Check sheet for the modelled part. Datum: model origin and axes. Units: mm. Face numbers are marked on the shaded views. A direction names the side the tool comes from. Round coordinates to 2 decimals unless told otherwise and drop trailing zeros. Loops run counter-clockwise (first coordinate to the right, second up) from the corner with the lowest first, then second, coordinate; pieces in that order, holes last. Notation, with made-up numbers: (-27, 22.25) - (-3, 22.25) arc R33 ccw to (-3, 56.25) - close; hole circle Ø4 at (2, 28). An arc over 180 degrees is marked (long way). Put each result on its own line as item: value.
```python
from build123d import *

# Parameters (mm, degrees)
SKETCH1_W           = 25
SKETCH1_H           = 16
BOSS_EXTRUDE1_DEPTH = 1
SKETCH2_W           = 20.55
SKETCH2_H           = 11.8
BOSS_EXTRUDE2_DEPTH = 2
FILLET1_R           = 2.5
FILLET2_R           = 0.5


with BuildPart() as part:
    # Sketch1 → Boss-Extrude1 (new body)
    with BuildSketch(Plane.XY):
        Rectangle(SKETCH1_W, SKETCH1_H)
    extrude(amount=-BOSS_EXTRUDE1_DEPTH)

    # Sketch2 → Boss-Extrude2 (add)
    with BuildSketch(Plane.XY):
        Rectangle(SKETCH2_W, SKETCH2_H)
    extrude(amount=BOSS_EXTRUDE2_DEPTH)

    # Fillet1
    fillet1_edges = [part.edges().sort_by_distance(p)[0] for p in [
        (10.275, -5.9, 1),
        (10.275, 5.9, 1),
        (-10.275, 5.9, 1),
        (-10.275, -5.9, 1),
        (12.5, -8, -0.5),
        (-12.5, -8, -0.5),
        (-12.5, 8, -0.5),
        (12.5, 8, -0.5),
    ]]
    fillet(fillet1_edges, radius=FILLET1_R)

    # Fillet2
    fillet2_edges = [part.edges().sort_by_distance(p)[0] for p in [
        (0, 5.9, 2),
        (10.275, 0, 2),
        (-10.275, 0, 2),
        (0, -5.9, 2),
        (9.542766953, -5.167766953, 2),
        (-9.542766953, -5.167766953, 2),
        (-9.542766953, 5.167766953, 2),
        (9.542766953, 5.167766953, 2),
    ]]
    fillet(fillet2_edges, radius=FILLET2_R)


solid = part.part
```
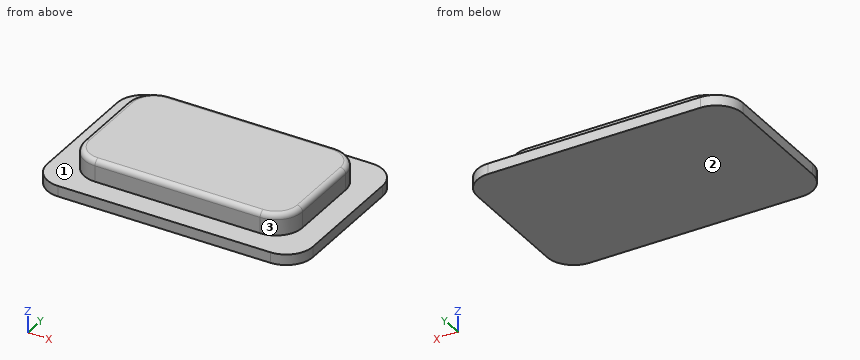
Item 1: Section check C-C on x = -3.25. Enter the section's corners in (y, z).
Filled sheet:
outline: (-8, -1) - (8, -1) - (8, 0) - (5.9, 0) - (5.9, 1.5) arc R0.5 ccw to (5.4, 2) - (-5.4, 2) arc R0.5 ccw to (-5.9, 1.5) - (-5.9, 0) - (-8, 0) - close
Item 2: Thickness scan on line 1 (Z direction, x = 11.25, y = 5.25); line 2 (X direction, y = 1.5, z = 0.3) (3 decimals); line 3 (Y direction, x = 0.75, z = 0.25). Record the ranges inside material, lowest first. Write a range as from..to.
Filled sheet:
line 1: -1..0
line 2: -10.275..10.275
line 3: -5.9..5.9
Item 3: Section check B-B on y = 0. Enter the section's corners in (x, z) (3 decimals), then the cut area to 3 significant figures.
Filled sheet:
outline: (-12.5, -1) - (12.5, -1) - (12.5, 0) - (10.275, 0) - (10.275, 1.5) arc R0.5 ccw to (9.775, 2) - (-9.775, 2) arc R0.5 ccw to (-10.275, 1.5) - (-10.275, 0) - (-12.5, 0) - close
area: 66.0 mm²
Item 4: Section check A-A on z = 0.4. Enter the section's corners in (x, y) (3 decimals).
Filled sheet:
outline: (-10.275, -3.4) arc R2.5 ccw to (-7.775, -5.9) - (7.775, -5.9) arc R2.5 ccw to (10.275, -3.4) - (10.275, 3.4) arc R2.5 ccw to (7.775, 5.9) - (-7.775, 5.9) arc R2.5 ccw to (-10.275, 3.4) - close
Item 5: Tool access check on the marked faces 1, 2 and 3. Record the directions out of +Z, -Z, +X, -X, +Y, -Y that give a thin tool (end or side, any length) a straight path to the whole face; none if there is none.
Filled sheet:
face 1: +Z
face 2: -Z, +X, -X, +Y, -Y
face 3: +Z, +X, -Y
Item 6: Go/stop test with flat-tipped pins: pin 1 (0.8 mm diameter, centred on y = -0.5, z = 1, fed in from -X) (3 decimals); pin 2 (0.8 mm diameter, centred on x = 1.5, z = 1, fed in from -Y); pin 3 (1.2 mm diameter, centred on x = 0, z = 1, fed in from +Y). Record where each tip stops, or that it passes through.
Filled sheet:
pin 1: x = -10.275
pin 2: y = -5.9
pin 3: y = 5.9
Item 7: Section check D-D on z = 1.75. Enter the section's corners in (x, y) (3 decimals), then the cut area to 3 significant figures.
Filled sheet:
outline: (-10.208, -3.4) arc R2.433 ccw to (-7.775, -5.833) - (7.775, -5.833) arc R2.433 ccw to (10.208, -3.4) - (10.208, 3.4) arc R2.433 ccw to (7.775, 5.833) - (-7.775, 5.833) arc R2.433 ccw to (-10.208, 3.4) - close
area: 233 mm²
